Model file for the job. Use its own axes, mm. A direction names the side the tool comes from. Give positions to 0.01 mm unless a question says otherwise; leave off trailing zeros. Write each loop counter-clockwise with the first axis right and the second up, starting at its lowest first coordinate (ties: lowest second). Pieces come first, ordered by that corner, then holes. Notation, with made-up numbers: (-21.5, -0.75) - (15.5, -0.75) arc R29 ccw to (15.5, 21.25) - close; hole circle Ø4 at (-2, 62). An arc over 180 degrees is marked (long way). Use CSV: the item, a comma, the result in double quotes.
from build123d import *

# Parameters (mm, degrees)
SKETCH_W            = 80
SKETCH_H            = 70
PAD_DEPTH           = 5
SKETCH001_R         = 1.8
HOLE_DEPTH          = 5.001
SKETCH005_R         = 2.25
HOLE003_DEPTH       = 5.001
SKETCH003_R         = 1.55
HOLE001_DEPTH       = 5.001
SKETCH002_R         = 5.5
HOLE002_DEPTH       = 25
POCKET_DEPTH        = 5.001
HOLE004_D           = 3.1
HOLE004_CBORE_D     = 3.5
HOLE004_CBORE_DEPTH = 2.5
POCKET001_DEPTH     = 4.4


with BuildPart() as part:
    # Sketch → Pad (new body)
    with BuildSketch(Plane.XY):
        Rectangle(SKETCH_W, SKETCH_H)
    extrude(amount=PAD_DEPTH)

    # Sketch001 (on Face6 of Pad) → Hole (cut, through all)
    with BuildSketch(Plane.XY.offset(5)):
        with Locations((-37.5, 25)):
            Circle(SKETCH001_R)
        with Locations((37.5, 25)):
            Circle(SKETCH001_R)
        with Locations((-37.5, -20)):
            Circle(SKETCH001_R)
        with Locations((37.5, -20)):
            Circle(SKETCH001_R)
    extrude(amount=-HOLE_DEPTH, mode=Mode.SUBTRACT)

    # Sketch005 (on Face5 of Hole) → Hole003 (cut, through all)
    with BuildSketch(Plane.XY.offset(5)):
        with Locations((-25, -30)):
            Circle(SKETCH005_R)
        with Locations((25, -30)):
            Circle(SKETCH005_R)
    extrude(amount=-HOLE003_DEPTH, mode=Mode.SUBTRACT)

    # Sketch003 (on Face5 of Hole003) → Hole001 (cut, through all)
    with BuildSketch(Plane.XY.offset(5)):
        with Locations((-16.255, 20)):
            Circle(SKETCH003_R)
        with Locations((16.255, 20)):
            Circle(SKETCH003_R)
        with Locations((-23.52, -7)):
            Circle(SKETCH003_R)
        with Locations((23.52, -7)):
            Circle(SKETCH003_R)
    extrude(amount=-HOLE001_DEPTH, mode=Mode.SUBTRACT)

    # Sketch002 (on Face5 of Hole001) → Hole002 (cut)
    with BuildSketch(Plane.XY.offset(5)):
        with Locations((-27, 7)):
            Circle(SKETCH002_R)
        with Locations((-27, 20)):
            Circle(SKETCH002_R)
    extrude(amount=-HOLE002_DEPTH, mode=Mode.SUBTRACT)

    # Sketch004 (on Face5 of Hole002) → Pocket (cut, through all)
    with BuildSketch(Plane.XY.offset(5)):
        with BuildLine():
            Line((-13.715, 23.94), (-13.715, 17.97))
            ThreePointArc((-13.715, 17.97), (-12.971051, 16.173949), (-11.175, 15.43))
            Line((-11.175, 15.43), (11.175, 15.43))
            ThreePointArc((11.175, 15.43), (12.971051, 16.173949), (13.715, 17.97))
            Line((13.715, 17.97), (13.715, 23.94))
            ThreePointArc((13.715, 23.94), (13.530477, 24.385477), (13.085, 24.57))
            Line((13.085, 24.57), (-13.085, 24.57))
            ThreePointArc((-13.085, 24.57), (-13.530477, 24.385477), (-13.715, 23.94))
        make_face()
        with BuildLine():
            Line((-21.26, -5.231721), (-20.431263, -9.931721))
            ThreePointArc((-20.431263, -9.931721), (-19.285496, -11.916249), (-17.132157, -12.7))
            Line((-17.132157, -12.7), (17.132157, -12.7))
            ThreePointArc((17.132157, -12.7), (19.285496, -11.916249), (20.431263, -9.931721))
            Line((20.431263, -9.931721), (21.26, -5.231721))
            ThreePointArc((21.26, -5.231721), (20.527143, -2.496662), (17.960894, -1.3))
            Line((17.960894, -1.3), (-17.960894, -1.3))
            ThreePointArc((-17.960894, -1.3), (-20.527143, -2.496662), (-21.26, -5.231721))
        make_face()
    extrude(amount=-POCKET_DEPTH, mode=Mode.SUBTRACT)

    # Hole004 (through all)
    with Locations(Plane(origin=(0, 0, 0), x_dir=(1, 0, 0), z_dir=(0, 0, -1))):
        with Locations((23.45, -20)):
            CounterBoreHole(HOLE004_D / 2, HOLE004_CBORE_D / 2, HOLE004_CBORE_DEPTH)

    # Sketch007 (on Face4 of Hole004) → Pocket001 (cut)
    with BuildSketch(Plane(origin=(0, 0, 0), x_dir=(1, 0, 0), z_dir=(0, 0, -1))):
        with BuildLine():
            Line((-18.4, -25.15), (18.4, -25.15))
            ThreePointArc((18.4, -25.15), (18.824264, -24.974264), (19, -24.55))
            Line((19, -24.55), (19, -16.85))
            ThreePointArc((21, -14.85), (19.585786, -15.435786), (19, -16.85))
            Line((21, -14.85), (24.7, -14.85))
            ThreePointArc((26.7, -16.85), (26.114214, -15.435786), (24.7, -14.85))
            Line((26.7, -16.85), (26.7, -23.15))
            ThreePointArc((26.7, -23.15), (27.285786, -24.564214), (28.7, -25.15))
            Line((28.7, -25.15), (33, -25.15))
            ThreePointArc((33, -25.15), (34.414214, -24.564214), (35, -23.15))
            Line((35, -23.15), (35, -1.525))
            ThreePointArc((35, -1.525), (34.414214, -0.110786), (33, 0.475))
            Line((33, 0.475), (28.75, 0.475))
            ThreePointArc((26.75, 2.475), (27.335786, 1.060786), (28.75, 0.475))
            Line((26.75, 2.475), (26.75, 11.525))
            ThreePointArc((28.75, 13.525), (27.335786, 12.939214), (26.75, 11.525))
            Line((33, 13.525), (28.75, 13.525))
            ThreePointArc((33, 13.525), (34.414214, 14.110786), (35, 15.525))
            Line((35, 22.775), (35, 15.525))
            ThreePointArc((35, 22.775), (34.414214, 24.189214), (33, 24.775))
            Line((-33, 24.775), (33, 24.775))
            ThreePointArc((-33, 24.775), (-34.414214, 24.189214), (-35, 22.775))
            Line((-35, 15.525), (-35, 22.775))
            ThreePointArc((-35, 15.525), (-34.414214, 14.110786), (-33, 13.525))
            Line((-28.75, 13.525), (-33, 13.525))
            ThreePointArc((-26.75, 11.525), (-27.335786, 12.939214), (-28.75, 13.525))
            Line((-26.75, 11.525), (-26.75, 1.075))
            ThreePointArc((-26.75, 1.075), (-26.574264, 0.650736), (-26.15, 0.475))
            Line((-26.15, 0.475), (-21, 0.475))
            ThreePointArc((-19, -1.525), (-19.585786, -0.110786), (-21, 0.475))
            Line((-19, -24.55), (-19, -1.525))
            ThreePointArc((-19, -24.55), (-18.824264, -24.974264), (-18.4, -25.15))
        make_face()
    extrude(amount=-POCKET001_DEPTH, mode=Mode.SUBTRACT)


solid = part.part
(1) Flat gauge pins, fed straight in: P1, Ø5, axis at x = -7.5, y = 12, coming from the -Z side; P2, Ø2.5, axis at x = -23.52, y = -7, coming from the -Z side. Where does each tip first touch, or does it go through?
Checked values:
P1,"stops at z = 4.4"
P2,"passes through"
(2) Wall check: probe 1 along Y at (x, z) = (-37.5, 2.3); probe 2 along Y at (x, z) = (5.5, 3.15) (3 decimals); probe 3 along X at (y, z) = (16, 3.05). Give the ranges that are in metal, low to high. Write a range as [from, to].
Checked values:
probe 1,"y = [-35, -21.8], [-18.2, 23.2], [26.8, 35]"
probe 2,"y = [-35, -24.775], [25.15, 35]"
probe 3,"x = [-40, -30.77], [-23.23, -19], [19.19, 26.51], [35, 40]"
(3) Saw through at D-D, the plane x = -4. List the corners of the cut face in (y, z) (3 decimals), then the cut area to 3 significant figures.
Checked values:
outline,"(-35, 0) - (-24.775, 0) - (-24.775, 4.4) - (-12.7, 4.4) - (-12.7, 5) - (-35, 5) - close; (-1.3, 4.4) - (15.43, 4.4) - (15.43, 5) - (-1.3, 5) - close; (24.57, 4.4) - (25.15, 4.4) - (25.15, 0) - (35, 0) - (35, 5) - (24.57, 5) - close"
area,"118 mm^2"
(4) Pull direction X, two halves, no side cores. Call faces 1 (the face through (19.26, -11.94, 4.7)), 2 (the face through (-1, -35, 2)): released by +X, released by -X, zero draft, split by the parting line, or undercut.
Checked values:
face 1,"undercut"
face 2,"zero draft"
(5) 3-axis set-ups, long thin cutter, end or side, ignore diameter. For faces 3 (the face through (17.1, 21.3, 4.7)), 4 (the face through (34.43, 0.126, 2.169)): which of +Z, -Z, +X, -X, +Y, -Y reach the whole face in a straight line?
Checked values:
face 3,"+Z, -Z"
face 4,"-Z"
(6) Saw through at C-C, the plane y = -20. List the corners of the cut face in (x, z).
Checked values:
outline,"(-40, 0) - (-39.3, 0) - (-39.3, 5) - (-40, 5) - close; (-35.7, 0) - (-35, 0) - (-35, 4.4) - (35, 4.4) - (35, 0) - (35.7, 0) - (35.7, 5) - (-35.7, 5) - close; (39.3, 0) - (40, 0) - (40, 5) - (39.3, 5) - close"
(7) Saw through at A-A, the plane y = 7. List the corners of the cut face in (x, z), then the cut area to 3 significant figures.
Checked values:
outline,"(-40, 0) - (-32.5, 0) - (-32.5, 5) - (-40, 5) - close; (-21.5, 0) - (-19, 0) - (-19, 4.4) - (35, 4.4) - (35, 0) - (40, 0) - (40, 5) - (-21.5, 5) - close"
area,"107 mm^2"
(8) Saw through at B-B, the plane x = 37.5. List the corners of the cut face in (y, z).
Checked values:
outline,"(-35, 0) - (-21.8, 0) - (-21.8, 5) - (-35, 5) - close; (-18.2, 0) - (23.2, 0) - (23.2, 5) - (-18.2, 5) - close; (26.8, 0) - (35, 0) - (35, 5) - (26.8, 5) - close"
